Input: part model. Units: mm. Frame: model coordinates. Round coordinates to 2 decimals unless told otherwise and drop trailing zeros. Answer in a Markdown table with one row per item. Add a question column.
Q1. Section A-A, the plane y = 0.7. Give the number of separate pieces and of enclosed holes in the cut face, and give its area (3 significant figures).
Q2. Ray query, L1, parallel to Z at x = 157.5, y = 0.5; L2, parallel to Z at x = 783, y = 0.4. Return the intervals inside material, ascending. Write a range as from..to.
Q3. Pin query (flat end, axial travel): pin 1 (9 mm diameter, centred on x = -22.5, z = 62.5, fed in from +Y). Return the tip coordinate at first contact, or that it passes through.
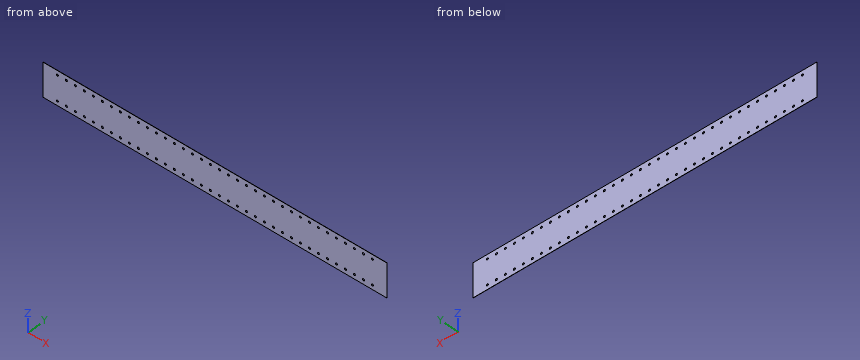
Autodesk Inventor part; units mm, degrees
ref_plane "YZ Plane" through (0, 0, 0) normal (1, 0, 0) x (0, 1, 0)
ref_plane "XZ Plane" through (0, 0, 0) normal (0, 1, 0) x (-1, 0, 0)
ref_plane "XY Plane" through (0, 0, 0) normal (0, 0, 1) x (1, 0, 0)
sketch "Skin Scheme" plane through (0, 0, 0) normal (0, 1, 0) x (-1, 0, 0)
  line L0 (909.5, -84.5) -> (-909.5, -84.5)
  line L1 (-909.5, -84.5) -> (-909.5, 84.5)
  line L2 (-909.5, 84.5) -> (909.5, 84.5)
  line L3 (909.5, 84.5) -> (909.5, -84.5)
  circle A0 centre (787.5, -62.5) radius 5
  circle A1 centre (742.5, -62.5) radius 5
  circle A2 centre (697.5, -62.5) radius 5
  circle A3 centre (652.5, -62.5) radius 5
  circle A4 centre (607.5, -62.5) radius 5
  circle A5 centre (562.5, -62.5) radius 5
  circle A6 centre (517.5, -62.5) radius 5
  circle A7 centre (472.5, -62.5) radius 5
  circle A8 centre (427.5, -62.5) radius 5
  circle A9 centre (382.5, -62.5) radius 5
  circle A10 centre (337.5, -62.5) radius 5
  circle A11 centre (292.5, -62.5) radius 5
  circle A12 centre (247.5, -62.5) radius 5
  circle A13 centre (202.5, -62.5) radius 5
  circle A14 centre (157.5, -62.5) radius 5
  circle A15 centre (112.5, -62.5) radius 5
  circle A16 centre (67.5, -62.5) radius 5
  circle A17 centre (22.5, -62.5) radius 5
  circle A18 centre (787.5, 62.5) radius 5
  circle A19 centre (742.5, 62.5) radius 5
  circle A20 centre (697.5, 62.5) radius 5
  circle A21 centre (652.5, 62.5) radius 5
  circle A22 centre (607.5, 62.5) radius 5
  circle A23 centre (562.5, 62.5) radius 5
  circle A24 centre (517.5, 62.5) radius 5
  circle A25 centre (472.5, 62.5) radius 5
  circle A26 centre (427.5, 62.5) radius 5
  circle A27 centre (382.5, 62.5) radius 5
  circle A28 centre (337.5, 62.5) radius 5
  circle A29 centre (292.5, 62.5) radius 5
  circle A30 centre (247.5, 62.5) radius 5
  circle A31 centre (202.5, 62.5) radius 5
  circle A32 centre (157.5, 62.5) radius 5
  circle A33 centre (112.5, 62.5) radius 5
  circle A34 centre (67.5, 62.5) radius 5
  circle A35 centre (22.5, 62.5) radius 5
  circle A36 centre (-22.5, -62.5) radius 5
  circle A37 centre (-22.5, 62.5) radius 5
  circle A38 centre (-67.5, -62.5) radius 5
  circle A39 centre (-67.5, 62.5) radius 5
  circle A40 centre (-112.5, -62.5) radius 5
  circle A41 centre (-112.5, 62.5) radius 5
  circle A42 centre (-157.5, -62.5) radius 5
  circle A43 centre (-157.5, 62.5) radius 5
  circle A44 centre (-202.5, -62.5) radius 5
  circle A45 centre (-202.5, 62.5) radius 5
  circle A46 centre (-247.5, -62.5) radius 5
  circle A47 centre (-247.5, 62.5) radius 5
  circle A48 centre (-292.5, -62.5) radius 5
  circle A49 centre (-292.5, 62.5) radius 5
  circle A50 centre (-337.5, -62.5) radius 5
  circle A51 centre (-337.5, 62.5) radius 5
  circle A52 centre (-382.5, -62.5) radius 5
  circle A53 centre (-382.5, 62.5) radius 5
  circle A54 centre (-427.5, -62.5) radius 5
  circle A55 centre (-427.5, 62.5) radius 5
  circle A56 centre (-472.5, -62.5) radius 5
  circle A57 centre (-472.5, 62.5) radius 5
  circle A58 centre (-517.5, -62.5) radius 5
  circle A59 centre (-517.5, 62.5) radius 5
  circle A60 centre (-562.5, -62.5) radius 5
  circle A61 centre (-562.5, 62.5) radius 5
  circle A62 centre (-607.5, -62.5) radius 5
  circle A63 centre (-607.5, 62.5) radius 5
  circle A64 centre (-652.5, -62.5) radius 5
  circle A65 centre (-652.5, 62.5) radius 5
  circle A66 centre (-697.5, -62.5) radius 5
  circle A67 centre (-697.5, 62.5) radius 5
  circle A68 centre (-742.5, -62.5) radius 5
  circle A69 centre (-742.5, 62.5) radius 5
  circle A70 centre (-787.5, -62.5) radius 5
  circle A71 centre (-787.5, 62.5) radius 5
  point P0 (0, 0)
  dimension "d0" = 1819
  dimension "d1" = 909.5
  dimension "d2" = 169
  dimension "d3" = 84.5
  dimension "d4" = 10
  dimension "d5" = 122
  dimension "d6" = 22
  dimension "d9" = 45
  dimension "d12" = 125
extrude "Skin Body" add sketch "Skin Scheme" along normal blind 1
sketch "End Cut Outline" plane through (0, 1, 0) normal (0, 1, 0) x (1, 0, 0)
  line L0 (-859.5, 94.5) -> (-919.5, 94.5)
  line L1 (-919.5, 94.5) -> (-919.5, -94.5)
  line L2 (-919.5, -94.5) -> (-859.5, -94.5)
  line L3 (-859.5, -94.5) -> (-859.5, 94.5)
  line L4 (909.5, 84.5) -> (-909.5, 84.5)
  line L5 (-909.5, -84.5) -> (909.5, -84.5)
  line L6 (-909.5, 84.5) -> (-909.5, -84.5)
  point P0 (0, 0)
  dimension "d19" = 10
  dimension "d20" = 10
  dimension "d21" = 10
  dimension "d22" = 50
extrude "End Cut" cut sketch "End Cut Outline" along normal through all both and the other way through all
mirror "End Cut Mirror" about plane through (0, 0, 0) normal (1, 0, 0) of "End Cut"
properties part number "Skin NPS 18 Internal" material "Rubber, Silicone"
Answer block:
| question | item | result |
|---|---|---|
| 1 | separate pieces | 1 |
| 1 | enclosed holes | 72 |
| 1 | area | 285,000 mm^2 |
| 2 | L1 | -84.5..-67.5, -57.5..57.5, 67.5..84.5 |
| 2 | L2 | -84.5..-64.68, -60.32..60.32, 64.68..84.5 |
| 3 | pin 1 | through |
